from build123d import *

# Parameters (mm, degrees)
SKETCH1_R                                       = 37.75
SKETCH1_R_2                                     = 9
BOSS_EXTRUDE1_DEPTH                             = 7
SKETCH1_5_R                                     = 39.75
SKETCH1_5_R_2                                   = 37.75
BOSS_EXTRUDE2_DEPTH                             = 40
CBORE_FOR_M3_SOCKET_HEAD_CAP_SCREW1_D           = 3.4
CBORE_FOR_M3_SOCKET_HEAD_CAP_SCREW1_CBORE_D     = 6.5
CBORE_FOR_M3_SOCKET_HEAD_CAP_SCREW1_CBORE_DEPTH = 3.4


with BuildPart() as part:
    # Sketch1 → Boss-Extrude1 (new body)
    with BuildSketch(Plane.XY):
        Circle(SKETCH1_R)
        Circle(SKETCH1_R_2, mode=Mode.SUBTRACT)
    extrude(amount=BOSS_EXTRUDE1_DEPTH)

    # Sketch1<5> → Boss-Extrude2 (add)
    with BuildSketch(Plane.XY):
        Circle(SKETCH1_5_R)
        Circle(SKETCH1_5_R_2, mode=Mode.SUBTRACT)
    extrude(amount=BOSS_EXTRUDE2_DEPTH)

    # CBORE for M3 Socket Head Cap Screw1 (through all)
    with Locations(Plane(origin=(-29.95, 0, 7), x_dir=(1, 0, 0), z_dir=(0, 0, 1))):
        with Locations((0, 0), (10.3, 0)):
            CounterBoreHole(CBORE_FOR_M3_SOCKET_HEAD_CAP_SCREW1_D / 2, CBORE_FOR_M3_SOCKET_HEAD_CAP_SCREW1_CBORE_D / 2, CBORE_FOR_M3_SOCKET_HEAD_CAP_SCREW1_CBORE_DEPTH)


solid = part.part
Design review of the part built by this model. Coordinates are the model's own, in mm. A direction names the side the tool comes from. Round coordinates to 2 decimals unless told otherwise and drop trailing zeros. Write each loop counter-clockwise with the first axis right and the second up, starting at its lowest first coordinate (ties: lowest second). Pieces come first, ordered by that corner, then holes. Notation, with made-up numbers: (-4.5, 79) - (54.5, 79) arc R29 cw to (54.5, 108) - close; hole circle Ø7 at (67.5, 33). An arc over 180 degrees is marked (long way). Use a Markdown table: item, result. Add a question column.
1. For faces 1 (the face through (8, -8, 7)), 2 (the face through (-21.2, -0.7, 1.8)), list the 3-axis set-ups (+Z, -Z, +X, -X, +Y, -Y) from which the entire face can be reached by the end or side of a thin tool; tool diameter is ignored.
2. Wall thickness on probe 1 along Y at (x, z) = (0, 28); probe 2 along X at (y, z) = (-1, 15); probe 3 along Z at (x, y) = (22.5, 4.5): over which ranges is each line inside the solid? List them lowest first.
3. Clearance check with flat-ended pins moving along their axes: pin 1 (12 mm diameter, centred on x = -22.5, y = 5.5, fed in from -Z); pin 2 (6 mm diameter, centred on x = 21, z = 4, fed in from +Y); pin 3 (3 mm diameter, centred on x = -30.5, y = 0, fed in from +Z); pin 4 (10 mm diameter, centred on x = -21.5, z = 18.5, fed in from -Y). State where each tip first meets the part, or that it passes through.
4. Mouldability with a two-part tool opening along X and no side actions: class faces 3 (the face through (-28.6, -1.4, 3.6)), 4 (the face through (15, -35, 40)), 5 (the face through (-5.175, 39.412, 19.72)), 6 (the face through (-16.55, 0.98, 5.32)) as +X half, -X half, draft (parallel to the pull), parting line (faces both ways), or undercut.
5. We need section C-C (y = 31.5). State the section outline as (x, z) points.
6. We need section D-D (z = 12). State the section outline as (x, y) points.
7. We need section B-B (y = 0). State the section outline as (x, z) points, then the cut area to 3 significant figures.
8. We need section A-A (x = 0). State the section outline as (y, z) points, then the cut area to 4 significant figures.
Output:
| question | item | result |
|---|---|---|
| 1 | face 1 | +Z |
| 1 | face 2 | +Z, -Z |
| 2 | probe 1 | y = -39.75 to -37.75, 37.75 to 39.75 |
| 2 | probe 2 | x = -39.74 to -37.74, 37.74 to 39.74 |
| 2 | probe 3 | z = 0 to 7 |
| 3 | pin 1 | stops at z = 0 |
| 3 | pin 2 | stops at y = 35.44 |
| 3 | pin 3 | stops at z = 3.6 |
| 3 | pin 4 | stops at y = -36.16 |
| 4 | face 3 | undercut |
| 4 | face 4 | draft |
| 4 | face 5 | parting line |
| 4 | face 6 | undercut |
| 5 | outline | (-24.24, 0) - (24.24, 0) - (24.24, 40) - (20.8, 40) - (20.8, 7) - (-20.8, 7) - (-20.8, 40) - (-24.24, 40) - close |
| 6 | outline | circle Ø79.5 at (0, 0); hole circle Ø75.5 at (0, 0) |
| 7 | outline | (-39.75, 0) - (-31.65, 0) - (-31.65, 3.6) - (-33.2, 3.6) - (-33.2, 7) - (-37.75, 7) - (-37.75, 40) - (-39.75, 40) - close; (-28.25, 0) - (-21.35, 0) - (-21.35, 3.6) - (-22.9, 3.6) - (-22.9, 7) - (-26.7, 7) - (-26.7, 3.6) - (-28.25, 3.6) - close; (-17.95, 0) - (-9, 0) - (-9, 7) - (-16.4, 7) - (-16.4, 3.6) - (-17.95, 3.6) - close; (9, 0) - (39.75, 0) - (39.75, 40) - (37.75, 40) - (37.75, 7) - (9, 7) - close |
| 7 | area | 494 mm2 |
| 8 | outline | (-39.75, 0) - (-9, 0) - (-9, 7) - (-37.75, 7) - (-37.75, 40) - (-39.75, 40) - close; (9, 0) - (39.75, 0) - (39.75, 40) - (37.75, 40) - (37.75, 7) - (9, 7) - close |
| 8 | area | 562.5 mm2 |
